Build history of the part. All positions in model axes, mm. Give positions to 0.01 mm unless a question says otherwise; leave off trailing zeros. Write each loop counter-clockwise with the first axis right and the second up, starting at its lowest first coordinate (ties: lowest second). Pieces come first, ordered by that corner, then holes.
from build123d import *

# Parameters (mm, degrees)
SKETCH_1_R      = 1.25
SKETCH_1_R_2    = 1
EXTRUDE_1_DEPTH = 2


with BuildPart() as part:
    # 草圖1 → 填料-伸長1 (new body)
    with BuildSketch(Plane.XY):
        with BuildLine():
            Line((-28.8, -32), (-28.8, -34))
            ThreePointArc((-28.8, -34), (-29.092893219, -34.707106781), (-29.8, -35))
            Line((-29.8, -35), (-31.8, -35))
            Line((-31.8, -35), (-31.8, -36))
            Line((-31.8, -36), (-31.8, -42))
            Line((-31.8, -42), (-31.8, -43))
            Line((-31.8, -43), (-30.8, -43))
            Line((-30.8, -43), (-26.8, -43))
            Line((-26.8, -43), (-25.8, -43))
            Line((-25.8, -43), (-25.8, -32))
            Line((-25.8, -32), (18.7, -32))
            Line((18.7, -32), (18.7, -43))
            Line((18.7, -43), (24.8, -43))
            Line((24.8, -43), (25.8, -43))
            Line((25.8, -43), (25.8, -42))
            Line((25.8, -42), (25.8, -36))
            Line((25.8, -36), (25.8, -35))
            Line((25.8, -35), (23.8, -35))
            ThreePointArc((23.8, -35), (23.092893219, -34.707106781), (22.8, -34))
            Line((22.8, -34), (22.8, -32))
            ThreePointArc((22.8, -32), (23.092893219, -31.292893219), (23.8, -31))
            Line((23.8, -31), (25.8, -31))
            Line((25.8, -31), (25.8, -18))
            Line((25.8, -18), (25.8, -17))
            Line((25.8, -17), (8.925896882, 6.428714091))
            ThreePointArc((8.925896882, 6.428714091), (0.800566406, 10.970829204), (-7.898074186, 7.656397596))
            Line((-7.898074186, 7.656397596), (-31.8, -17))
            Line((-31.8, -17), (-31.8, -18))
            Line((-31.8, -18), (-31.8, -31))
            Line((-31.8, -31), (-29.8, -31))
            ThreePointArc((-29.8, -31), (-29.092893219, -31.292893219), (-28.8, -32))
        make_face()
        Circle(SKETCH_1_R, mode=Mode.SUBTRACT)
        with Locations((-19.05, -21)):
            Circle(SKETCH_1_R_2, mode=Mode.SUBTRACT)
        with Locations((-11.05, -21)):
            Circle(SKETCH_1_R_2, mode=Mode.SUBTRACT)
        with Locations((4.95, -21)):
            Circle(SKETCH_1_R_2, mode=Mode.SUBTRACT)
        with Locations((12.95, -21)):
            Circle(SKETCH_1_R_2, mode=Mode.SUBTRACT)
        with Locations((-27.8, -29)):
            Circle(SKETCH_1_R_2, mode=Mode.SUBTRACT)
        with Locations((-27.8, -37)):
            Circle(SKETCH_1_R_2, mode=Mode.SUBTRACT)
        with Locations(Location((21.8, -37, 0), (0, 0, 180))):
            Circle(SKETCH_1_R_2, mode=Mode.SUBTRACT)
        with Locations(Location((21.8, -29, 0), (0, 0, 180))):
            Circle(SKETCH_1_R_2, mode=Mode.SUBTRACT)
        with Locations((-7.05, -21)):
            Circle(SKETCH_1_R_2, mode=Mode.SUBTRACT)
        with Locations((0.95, -21)):
            Circle(SKETCH_1_R_2, mode=Mode.SUBTRACT)
    extrude(amount=EXTRUDE_1_DEPTH)


solid = part.part
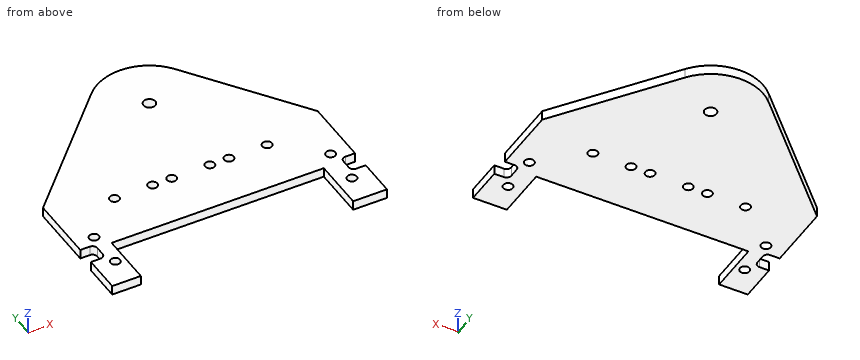
1. Saw through at B-B on y = -37. Give the cut face in (x, z).
2. Saw through at A-A on z = 1.2. Count the separate pieces of the cut face and the enclosed holes in it, plus the area to 3 significant figures.
3. Saw through at C-C on x = 21.8. Give the cut face in (y, z), plus the area to 3 significant figures.
4. Drop flat-ended pins along their axis: pin 1 (5 mm diameter, centred on x = 0.5, y = 0.5, fed in from -Z); pin 2 (1 mm diameter, centred on x = 14.5, z = 1.5, fed in from +Y); pin 3 (1 mm diameter, centred on x = 9.5, z = 1, fed in from +Y). Give the stop position or say it passes through.
5. Saw through at D-D on y = -21. Give the cut face in (x, z).
6. Drill centre lines: line 1 along Y through (x, z) = (-27.8, 0.4); line 2 along Y through (x, z) = (-19, 0.5); line 3 along Y through (x, z) = (21.8, 1.05). Where is each one in solid material? Low to high.
Outcome:
1. outline: (-31.8, 0) - (-28.8, 0) - (-28.8, 2) - (-31.8, 2) - close; (-26.8, 0) - (-25.8, 0) - (-25.8, 2) - (-26.8, 2) - close; (18.7, 0) - (20.8, 0) - (20.8, 2) - (18.7, 2) - close; (22.8, 0) - (25.8, 0) - (25.8, 2) - (22.8, 2) - close
2. separate pieces: 1
2. enclosed holes: 11
2. area: 1,890 mm2
3. outline: (-43, 0) - (-38, 0) - (-38, 2) - (-43, 2) - close; (-36, 0) - (-30, 0) - (-30, 2) - (-36, 2) - close; (-28, 0) - (-11.45, 0) - (-11.45, 2) - (-28, 2) - close
3. area: 55.1 mm2
4. pin 1: stops at z = 0
4. pin 2: stops at y = -0.62
4. pin 3: stops at y = 6.33
5. outline: (-31.8, 0) - (-20.05, 0) - (-20.05, 2) - (-31.8, 2) - close; (-18.05, 0) - (-12.05, 0) - (-12.05, 2) - (-18.05, 2) - close; (-10.05, 0) - (-8.05, 0) - (-8.05, 2) - (-10.05, 2) - close; (-6.05, 0) - (-0.05, 0) - (-0.05, 2) - (-6.05, 2) - close; (1.95, 0) - (3.95, 0) - (3.95, 2) - (1.95, 2) - close; (5.95, 0) - (11.95, 0) - (11.95, 2) - (5.95, 2) - close; (13.95, 0) - (25.8, 0) - (25.8, 2) - (13.95, 2) - close
6. line 1: y = -43 to -38, -36 to -30, -28 to -12.87
6. line 2: y = -32 to -22, -20 to -3.8
6. line 3: y = -43 to -38, -36 to -30, -28 to -11.45
